Part print with two shaded views. Sizes in mm from the minimum x, y, z corner. A direction names the side the tool comes from. Coordinates: 2 decimals unless noted, no trailing zeros. Loops run counter-clockwise (first coordinate to the right, second up) from the corner with the lowest first, then second, coordinate; pieces in that order, holes last. Notation, with made-up numbers: (75, -21) -> (103, -21) arc R19 cw to (103, 2) -> close; hole circle Ø7 at (-39.75, 26). An arc over 180 degrees is marked (long way). Return JSON: item names as keys, results as strings. Group by question number.
(1) Saw through at B-B on y = 1.5. Write the cut outline in (x, z) (3 decimals).
(2) Flat gauge pins, fed straight in: pin 1 Ø2 at (x, y) = (4.5, 2.5) entering from -Z; pin 2 Ø1 at (y, z) = (1, 1.5) entering from +X; pin 3 Ø1.5 at (y, z) = (2.5, 11) entering from +X. Where does each tip first touch, or does it go through?
(3) Mould opens along Z. For the marked faces 3, 4, 5 and 6 say: pulls with the +Z half, pulls with the -Z half, needs draft (parallel to the pull), parting line crosses it, or undercut.
(4) Probe L1, parallel to Z at x = 6.35, y = 1 (3 decimals); L2, parallel to X at y = 4.75, z = 6.5; L3, parallel to Z at x = 5.5, y = 1.75. List the from-to ranges inside material, lowest first.
(5) Tool access for the marked faces 1 and 2: list every direction of +Z, -Z, +X, -X, +Y, -Y with a clear straight run to the whole face (end or side of a thin tool).
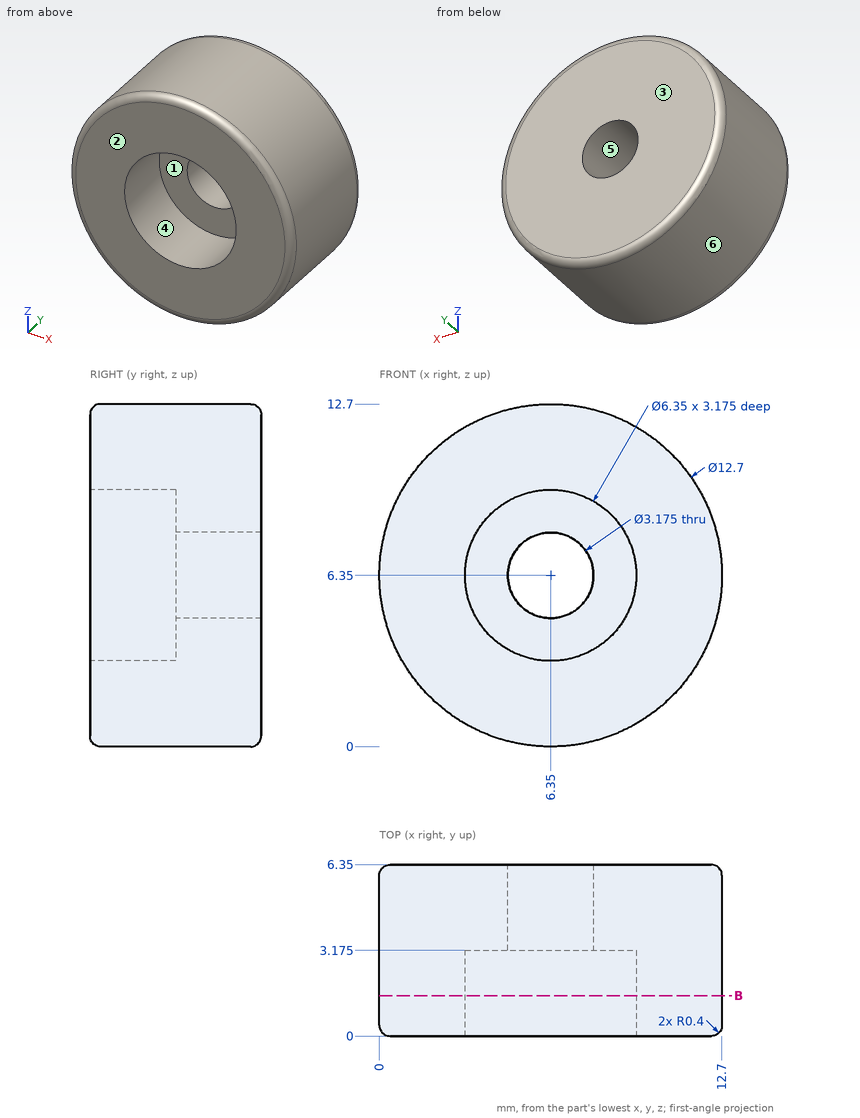
Geometry results:
{
 "1": {"outline": "circle Ø12.7 at (6.35, 6.35); hole circle Ø6.35 at (6.35, 6.35)"},
 "2": {"pin 1": "z = 0.06", "pin 2": "x = 10.98", "pin 3": "x = 11.36"},
 "3": {"face 3": "needs draft", "face 4": "undercut", "face 5": "undercut", "face 6": "parting line crosses it"},
 "4": {"L1": "0 to 3.175, 9.525 to 12.7", "L2": "0 to 4.77, 7.93 to 12.7", "L3": "0.06 to 3.29, 9.41 to 12.64"},
 "5": {"face 1": "-Y", "face 2": "+Z, -Z, +X, -X, -Y"}
}
